The model under review builds one solid part; all positions refer to its coordinate system, in mm. A direction names the side the tool comes from. Give positions to 0.01 mm unless a question says otherwise; leave off trailing zeros. Order: outer loops, then holes, each group sorted by start corner. A loop starts at its lowest first (then second) coordinate and runs counter-clockwise, first axis right, second up. Notation, with made-up numbers: (32.5, 81) -> (76.5, 81) arc R17 ccw to (76.5, 104) -> close; hole circle Ø8 at (21.5, 3). An arc over 180 degrees is marked (long way). Use one line per item in the form item = value.
Autodesk Inventor part; units mm, degrees
ref_plane "IDS_WORKPLANE{1}" through (-4.826, 0, 0) normal (1, 0, 0) x (0, 0, -1)
ref_plane "Work Plane2" through (-2.413, 0, 0) normal (0, 0, -1) x (1, 0, 0)
ref_plane "YZ Plane" through (0, 0, 0) normal (1, 0, 0) x (0, 1, 0)
sketch "Sketch1" plane through (0, 0, 0) normal (0, 0, 1) x (1, 0, 0)
  line L0 (-4.826, 0) -> (57.15, 0)
  line L1 (57.15, 0) -> (57.15, 2.413)
  line L2 (57.15, 2.413) -> (0, 2.413)
  line L3 (0, 2.413) -> (0, 3.9624)
  line L4 (-19.3761, 0) -> (69.9044, 0)
  line L5 (0, -0.7925) -> (0, 4.7549)
  line L6 (0, 3.9624) -> (-4.826, 3.9624)
  line L7 (-4.826, 0) -> (-4.826, 3.9624)
  arc A0 (-1.9085, 0) -> (-2.54, 2.3566) centre (-6.6218, 0) ccw
  line L8 (-4.826, 2.3566) -> (-2.54, 2.3566)
  line L9 (12.7, 2.413) -> (0, 2.413) construction
  dimension "d0" = 57.15
  dimension "d1" = 4.826
  dimension "d2" = 4.826
  dimension "d5" = 7.9248
  dimension "d13" = 4.7132
  dimension "d14" = 4.7132
  dimension "d15" = 2.286
revolve "Body" add sketch "Sketch1" angle 360 about axis through (-4.826, 0, 0) along (1, 0, 0) contours A0 L8 L7 L6 L3 L5 L0 | L5 L2 L1 L0
ref_plane "IDS_WORKPLANE{1}" through (-4.826, 0, 0) normal (1, 0, 0) x (0, 0, -1)
sketch "Sketch2" plane through (-4.826, 0, 0) normal (1, 0, 0) x (0, 0, -1)
  line L0 (0, -5.5474) -> (0, 5.5474)
  line L1 (5.7744, 0) -> (-5.5852, 0)
  circle A0 centre (0, 0) radius 3.9624
  line L2 (2.3026, 0.5017) -> (1.9783, 0.5016)
  line L3 (0, 0) -> (2.3026, 0.5017) construction
  line L4 (0, 0) -> (4.1516, 3.7764) construction
  line L5 (0, 0) -> (0.7169, 2.2449) construction
  line L6 (0, 0) -> (1.1783, 2.0409) construction
  line L7 (0.7169, 2.2449) -> (0.5547, 1.9641)
  line L8 (1.5857, 1.7433) -> (1.4236, 1.4624)
  line L9 (0, 0) -> (1.5857, 1.7433) construction
  arc A1 (2.0409, 0) -> (1.9783, 0.5016) centre (0, 0) ccw
  arc A2 (1.4236, 1.4624) -> (0.5547, 1.9641) centre (0, 0) ccw
  arc A3 (2.3566, 0) -> (2.3026, 0.5017) centre (0, 0) ccw
  arc A4 (1.5857, 1.7433) -> (0.7169, 2.2449) centre (0, 0) ccw
  arc A5 (2.3026, 0.5017) -> (1.3897, 1.9032) centre (0, 0) ccw construction
  arc A6 (1.9783, 0.5016) -> (1.4236, 1.4624) centre (0, 0) ccw construction
  line L10 (2.3026, -0.5017) -> (1.9783, -0.5016)
  line L11 (0.7169, -2.2449) -> (0.5547, -1.9641)
  line L12 (1.5857, -1.7433) -> (1.4236, -1.4624)
  arc A7 (1.9783, -0.5016) -> (2.0409, 0) centre (0, 0) ccw
  arc A8 (0.5547, -1.9641) -> (1.4236, -1.4624) centre (0, 0) ccw
  arc A9 (2.3026, -0.5017) -> (2.3566, 0) centre (0, 0) ccw
  arc A10 (0.7169, -2.2449) -> (1.5857, -1.7433) centre (0, 0) ccw
  line L13 (-2.3026, 0.5017) -> (-1.9783, 0.5016)
  line L14 (-0.7169, 2.2449) -> (-0.5547, 1.9641)
  line L15 (-1.5857, 1.7433) -> (-1.4236, 1.4624)
  arc A11 (-1.9783, 0.5016) -> (-2.0409, 0) centre (0, 0) ccw
  arc A12 (-0.5547, 1.9641) -> (-1.4236, 1.4624) centre (0, 0) ccw
  arc A13 (-2.3026, 0.5017) -> (-2.3566, 0) centre (0, 0) ccw
  arc A14 (-0.7169, 2.2449) -> (-1.5857, 1.7433) centre (0, 0) ccw
  line L16 (-0.7169, -2.2449) -> (-0.5547, -1.9641)
  arc A15 (-1.4236, -1.4624) -> (-0.5547, -1.9641) centre (0, 0) ccw
  line L17 (-1.5857, -1.7433) -> (-1.4236, -1.4624)
  arc A16 (-1.5857, -1.7433) -> (-0.7169, -2.2449) centre (0, 0) ccw
  arc A17 (-2.0409, 0) -> (-1.9783, -0.5016) centre (0, 0) ccw
  line L18 (-2.3026, -0.5017) -> (-1.9783, -0.5016)
  arc A18 (-2.3566, 0) -> (-2.3026, -0.5017) centre (0, 0) ccw
  point P0 (1.1783, -2.0409)
  point P1 (-1.1783, 2.0409)
  point P2 (-1.1783, -2.0409)
  dimension "d19" = 0.5017
  dimension "d20" = 1.0033
  dimension "d21" = 35.419
  dimension "d22" = 4.7132
  dimension "d23" = 4.0818
extrude "Slot" add sketch "Sketch2" along normal up to next contours A1 L2 A3 L1 | L1 A9 L10 A7 | A17 L18 A18 L1 | L1 A13 L13 A11 | A4 L8 A2 L7 | L11 A8 L12 A10 | L14 A12 L15 A14 | A16 L17 A15 L16
fillet "Fillet1" radius 0.4572 1 edges at (-4.826, -3.9624, 0)
thread "Thread"
chamfer "Chamfer1" distance 0.6299 distance2 0.6299 1 edges at (57.15, -2.413, 0) measured on face at (57.15, -0.9495, -0.1286)
ref_plane "Work Plane2" through (-2.413, 0, 0) normal (0, 0, -1) x (1, 0, 0)
equation "\"d19\" = 0.5 * SBR"
equation "\"d20\" = SBR"
equation "\"d22\" = 1.1547 * SW"
equation "\"d23\" = SW"
equation "\"d17\" = INTI"
equation "\"d24\" = RR"
equation "\"d6\" = GEL"
equation "\"d9\" = -0.5 * SPD + 0.5 * NND"
equation "\"d10\" = GUL"
equation "\"d0\" = NLG"
equation "\"d1\" = KOH"
equation "\"d2\" = NND"
equation "\"d5\" = KOD"
equation "\"d13\" = 1.1547 * SW"
equation "\"d14\" = 1.1547 * SW"
equation "\"d15\" = INTI"
equation "\"NND\" = 4.826"
equation "\"NLG\" = 57.15"
equation "\"GEL\" = 22.098"
equation "\"KOD\" = 7.9248"
equation "\"KOH\" = 4.826"
equation "\"SPD\" = GD1"
equation "\"GUL\" = 0.62992"
equation "\"SBR\" = 1.0033"
equation "\"INTI\" = 2.286"
equation "\"d11\" = -KOH"
equation "\"SW\" = 4.08178"
equation "\"d16\" = 1.1547 * SW"
equation "\"d18\" = SW"
equation "\"RR\" = 0.4572"
equation "\"TOA\" = 30deg"
equation "\"GD1\" = 3.56616"
equation "\"THREADDIA\" = 4.826"
equation "\"BDM\" = NND"
equation "\"GD\" = NND"
equation "\"GAL\" = 2.64592"
equation "\"E0\" = 4.71678"
properties part number "ANSI B18.3 - 10-24 UNC - 2.25" material "Steel, Mild"
1. Add section A-A on x = 34.5. Give the boundary of the cut face in (y, z), then the cut area to 3 significant figures.
Values:
outline = circle Ø4.83 at (0, 0)
area = 18.3 mm^2
2. The part is to be moulded in two halves that separate along Y. For faces 1 (the face through (57.15, 0, 0)), 2 (the face through (-3.667, -2.357, 0.01)), 3 (the face through (-2.21, -0.52, -3.93)), say which applies: +Y half, -Y half, draft (parallel to the pull), parting line (faces both ways), or undercut.
Values:
face_1 = draft
face_2 = undercut
face_3 = parting line
3. For pin 1 Ø1 at (x, y) = (13, 2) entering from -Z; pin 2 Ø4 at (x, y) = (8.5, 0.5) entering from -Z, all flat-tipped, find the tip position at first contact; note any pin that passes through.
Values:
pin_1 = -1.89
pin_2 = -2.41
4. For L1, parallel to Y at x = 12.5, z = -0.75; L2, parallel to Y at x = 39.5, z = 0.5; L3, parallel to X at y = -3, z = -0.25, list the stretches that pass through material, from the lowest coordinate up.
Values:
L1 = -2.29 to 2.29
L2 = -2.36 to 2.36
L3 = -4.83 to 0
5. Tool access review of faces 4 (the face through (27.864, -1.915, 1.468)), 5 (the face through (-4.826, 0, -2.3)): name each direction out of +Z, -Z, +X, -X, +Y, -Y from which nothing blocks a thin tool from reaching the whole face with its end or side.
Values:
face_4 = +X
face_5 = +Z, -Z, -X, +Y, -Y
